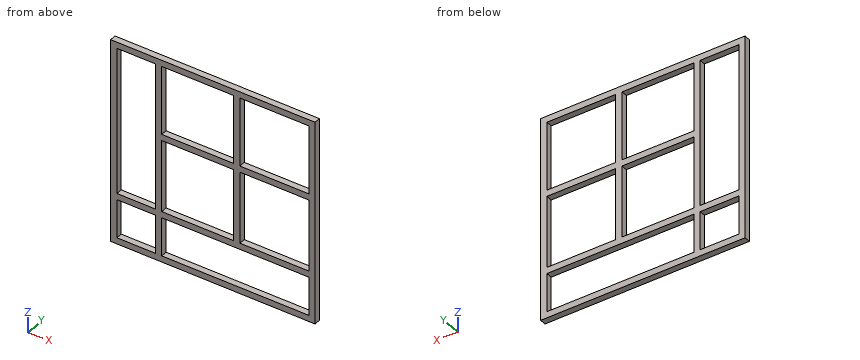
```python
from build123d import *

# Parameters (mm, degrees)
SKETCH2_W           = 426.044
SKETCH2_H           = 426.044
SKETCH2_W_2         = 80.467
SKETCH2_H_2         = 306.511
SKETCH2_H_3         = 80.467
SKETCH2_W_3         = 143.489
SKETCH2_H_4         = 143.489
SKETCH2_W_4         = 306.511
SKETCH2_W_5         = 150
SKETCH2_H_5         = 150
BOSS_EXTRUDE1_DEPTH = 13.022


with BuildPart() as part:
    # Sketch2 → Boss-Extrude1 (new body)
    with BuildSketch(Plane(origin=(0, 0, 0), x_dir=(1, 0, 0), z_dir=(0, 1, 0))):
        with Locations((213.022, 213.022)):
            Rectangle(SKETCH2_W, SKETCH2_H)
        with Locations((53.2555, 166.2775)):
            Rectangle(SKETCH2_W_2, SKETCH2_H_2, mode=Mode.SUBTRACT)
        with Locations((53.2555, 372.7885)):
            Rectangle(SKETCH2_W_2, SKETCH2_H_3, mode=Mode.SUBTRACT)
        with Locations((341.2775, 84.7665)):
            Rectangle(SKETCH2_W_3, SKETCH2_H_4, mode=Mode.SUBTRACT)
        with Locations((259.7665, 372.7885)):
            Rectangle(SKETCH2_W_4, SKETCH2_H_3, mode=Mode.SUBTRACT)
        with Locations((181.511, 84.7665)):
            Rectangle(SKETCH2_W_5, SKETCH2_H_4, mode=Mode.SUBTRACT)
        with Locations((181.511, 244.533)):
            Rectangle(SKETCH2_W_5, SKETCH2_H_5, mode=Mode.SUBTRACT)
        with Locations((341.2775, 244.533)):
            Rectangle(SKETCH2_W_3, SKETCH2_H_5, mode=Mode.SUBTRACT)
    extrude(amount=BOSS_EXTRUDE1_DEPTH)


solid = part.part
```
The listing builds one solid part. Answer for the finished solid, in the listing's coordinates (mm). Coordinates: 2 decimals unless noted, no trailing zeros. Write each loop counter-clockwise with the first axis right and the second up, starting at its lowest first coordinate (ties: lowest second). Pieces come first, ordered by that corner, then holes. Notation, with made-up numbers: (38.5, -13) - (43.5, -13) arc R20 ccw to (43.5, 22) - close; hole circle Ø7 at (65, 43.25). An arc over 180 degrees is marked (long way). One line per item, written item: value.
1) Consider line 1 along Z through (x, y) = (218.5, 9) (3 decimals); line 2 along X through (y, z) = (4.25, -269); line 3 along X through (y, z) = (8, -371). Determine where each line is inside the solid, lowest interval first. Write a range as from..to.
Geometry check:
line 1: z = -426.044..-413.022, -332.555..-319.533, -169.533..-156.511, -13.022..0
line 2: x = 0..13.02, 93.49..106.51, 256.51..269.53, 413.02..426.04
line 3: x = 0..13.02, 93.49..106.51, 413.02..426.04
2) Find section B-B (y = 4). Count the separate pieces of the cut face and the enclosed holes in it, and give its area (3 significant figures).
Geometry check:
separate pieces: 1
enclosed holes: 7
area: 39,600 mm2
3) Find section D-D (z = -147). Give the vertices of the cut face in (x, y), and give its area (3 significant figures).
Geometry check:
outline: (0, 0) - (13.02, 0) - (13.02, 13.02) - (0, 13.02) - close; (93.49, 0) - (106.51, 0) - (106.51, 13.02) - (93.49, 13.02) - close; (256.51, 0) - (269.53, 0) - (269.53, 13.02) - (256.51, 13.02) - close; (413.02, 0) - (426.04, 0) - (426.04, 13.02) - (413.02, 13.02) - close
area: 678 mm2
4) Find section A-A (z = -362). Give the vertices of the cut face in (x, y).
Geometry check:
outline: (0, 0) - (13.02, 0) - (13.02, 13.02) - (0, 13.02) - close; (93.49, 0) - (106.51, 0) - (106.51, 13.02) - (93.49, 13.02) - close; (413.02, 0) - (426.04, 0) - (426.04, 13.02) - (413.02, 13.02) - close
5) Find section C-C (x = 184). Give the vertices of the cut face in (y, z) (3 decimals), and give its area (3 significant figures).
Geometry check:
outline: (0, -426.044) - (13.022, -426.044) - (13.022, -413.022) - (0, -413.022) - close; (0, -332.555) - (13.022, -332.555) - (13.022, -319.533) - (0, -319.533) - close; (0, -169.533) - (13.022, -169.533) - (13.022, -156.511) - (0, -156.511) - close; (0, -13.022) - (13.022, -13.022) - (13.022, 0) - (0, 0) - close
area: 678 mm2
